```python
from build123d import *

# Parameters (mm, degrees)
F1_DEPTH = 50.8


with BuildPart() as f1:
    # F0 (on Top) → F1 (new body)
    with BuildSketch(Plane.XY):
        with BuildLine():
            ThreePointArc((-1.5875, 4.4901280605), (-2.749630657, -3.8885649667), (4.7625, 0))
            ThreePointArc((4.7625, 0), (3.8885649667, 2.749630657), (1.5875, 4.4901280605))
            Line((1.5875, 4.4901280605), (-1.5875, 4.4901280605))
        make_face()
        with BuildLine():
            Line((-1.5875, 4.4901280605), (1.5875, 4.4901280605))
            ThreePointArc((1.5875, 4.4901280605), (0, 4.7625), (-1.5875, 4.4901280605))
        make_face()
        with BuildLine():
            ThreePointArc((-1.5875, 4.4901280605), (0, 4.7625), (1.5875, 4.4901280605))
            Line((1.5875, 4.4901280605), (1.5875, 9.5701280605))
            Line((1.5875, 9.5701280605), (-1.5875, 9.5701280605))
            Line((-1.5875, 9.5701280605), (-1.5875, 4.4901280605))
        make_face()
    extrude(amount=F1_DEPTH)


solid = f1.part
```
Verification items for the finished model (mm, model axes). A direction names the side the tool comes from. Coordinates: 2 decimals unless noted, no trailing zeros. Order: outer loops, then holes, each group sorted by start corner. A loop starts at its lowest first (then second) coordinate and runs counter-clockwise, first axis right, second up. Notation, with made-up numbers: (80, 38.5) -> (91, 38.5) arc R31 cw to (91, 74.5) -> close; hole circle Ø10 at (-36.5, 59.5). An arc over 180 degrees is marked (long way). Put each result on its own line as item: value. Start each with the question number.
1) Tool access check on faces 1 (the flat face through (1.588, 7, 25)), 2 (the flat face through (0, 1, 0)). Record the directions out of +Z, -Z, +X, -X, +Y, -Y that give a thin tool (end or side, any length) a straight path to the whole face; none if there is none.
2) Cross-section at A-A (z = 35.5). Enter the section's corners in (x, y) (1 decimal), plus the area to 3 significant figures.
3) Cross-section at B-B (y = 8.5). Enter the section's corners in (x, z).
4) Release check for a two-part mould opening along Y. For faces 3 (the flat face through (-1.588, 7, 25)), 4 (the flat face through (0, 9.57, 25)) record: pulls with the +Y half, pulls with the -Y half, needs draft (parallel to the pull), parting line crosses it, or undercut.
5) Cross-section at C-C (x = 4). Enter the section's corners in (y, z).
6) Go/stop test with flat-tipped pins: pin 1 (2 mm diameter, centred on y = 5, z = 25, fed in from +X); pin 2 (4 mm diameter, centred on y = 8, z = 19.5, fed in from +X); pin 3 (3 mm diameter, centred on y = 3, z = 5, fed in from -X). Record where each tip stops, or that it passes through.
7) Material ranges on L1, parallel to X at y = 7, z = 33; L2, parallel to Y at x = 0.25, z = 34; L3, parallel to X at y = -0.5, z = 38, recorded low to high.
Geometry check:
1. face 1: +Z, -Z, +X, +Y
1. face 2: -Z, +X, -X, +Y, -Y
2. outline: (-1.6, 4.5) arc R4.8 ccw (long way) to (1.6, 4.5) -> (1.6, 9.6) -> (-1.6, 9.6) -> close
2. area: 86.8 mm^2
3. outline: (-1.59, 0) -> (1.59, 0) -> (1.59, 50.8) -> (-1.59, 50.8) -> close
4. face 3: needs draft
4. face 4: pulls with the +Y half
5. outline: (-2.58, 0) -> (2.58, 0) -> (2.58, 50.8) -> (-2.58, 50.8) -> close
6. pin 1: stops at x = 2.58
6. pin 2: stops at x = 1.59
6. pin 3: stops at x = -4.52
7. L1: x = -1.59 to 1.59
7. L2: y = -4.76 to 9.57
7. L3: x = -4.74 to 4.74
